from build123d import *

# Parameters (mm, degrees)
SKETCH1_R               = 1.05
SKETCH1_R_2             = 2.35
BOSS_EXTRUDE1_DEPTH     = 3
ENL_V_MAT_EXTRU_1_DEPTH = 1.5
ESQUISSE3_R             = 0.5
ESQUISSE3_R_2           = 3.75
ENL_V_MAT_EXTRU_7_DEPTH = 22.478826932


with BuildPart() as part:
    # Sketch1 → Boss-Extrude1 (new body)
    with BuildSketch(Plane(origin=(0, 0, 0), x_dir=(1, 0, 0), z_dir=(0, 1, 0))):
        with BuildLine():
            Line((15.3, 15), (12.3, 15))
            ThreePointArc((12.3, 15), (3.958234572, 13.40032808), (-3.2, 8.828273999))
            ThreePointArc((-3.2, 8.828273999), (-7, 0), (-3.2, -8.828273999))
            ThreePointArc((-3.2, -8.828273999), (3.958234572, -13.40032808), (12.3, -15))
            Line((12.3, -15), (15.3, -15))
            Line((15.3, -15), (15.3, 15))
        make_face()
        with Locations(Location((13.8, -10, 0), (0, 0, 270))):
            Circle(SKETCH1_R, mode=Mode.SUBTRACT)
        with Locations(Location((13.8, 10, 0), (0, 0, 270))):
            Circle(SKETCH1_R, mode=Mode.SUBTRACT)
        with Locations(Location((0, 0, 0), (0, 0, 270))):
            Circle(SKETCH1_R_2, mode=Mode.SUBTRACT)
    extrude(amount=-BOSS_EXTRUDE1_DEPTH)

    # Esquisse1 → Enlèv. mat.-Extru.1 (cut)
    with BuildSketch(Plane(origin=(0, 0, 0), x_dir=(1, 0, 0), z_dir=(0, 1, 0))):
        with BuildLine():
            Line((2.494493937, -2.8), (14.131406802, -1.932309126))
            add(Edge.make_bspline(
                [(14.131406802, -1.932309126), (14.497286128, -1.904835216), (14.827491954, -1.746052706), (15.157338026, -1.587443187), (15.407154881, -1.318584734), (15.656200737, -1.050556048), (15.790562016, -0.709168668), (15.92490372, -0.367831024), (15.925, 0), (15.925095847, 0.366175279), (15.791018176, 0.708007672), (15.657374187, 1.048734388), (15.407835717, 1.317851242), (15.159067388, 1.586137532), (14.828615817, 1.74551148), (14.498449498, 1.904747853), (14.131406802, 1.932309126)],
                knots=[0, 0, 0, 0.125, 0.125, 0.25, 0.25, 0.375, 0.375, 0.5, 0.5, 0.625, 0.625, 0.75, 0.75, 0.875, 0.875, 1, 1, 1], degree=2))
            Line((14.131406802, 1.932309126), (2.494493937, 2.8))
            ThreePointArc((2.494493937, 2.8), (-3.75, 0), (2.494493937, -2.8))
        make_face()
    extrude(amount=-ENL_V_MAT_EXTRU_1_DEPTH, mode=Mode.SUBTRACT)

    # Esquisse3 → Enlèv. mat.-Extru.7 (cut, through all)
    with BuildSketch(Plane(origin=(0, -1.5, 0), x_dir=(1, 0, 0), z_dir=(0, 1, 0))):
        with Locations(Location((4.9, 0, 0), (0, 0, 270))):
            Circle(ESQUISSE3_R)
        with Locations(Location((6.9, 0, 0), (0, 0, 270))):
            Circle(ESQUISSE3_R)
        with Locations(Location((8.9, 0, 0), (0, 0, 270))):
            Circle(ESQUISSE3_R)
        with Locations(Location((10.9, 0, 0), (0, 0, 270))):
            Circle(ESQUISSE3_R)
        with Locations(Location((12.9, 0, 0), (0, 0, 270))):
            Circle(ESQUISSE3_R)
        with Locations(Location((0, 0, 0), (0, 0, 270))):
            Circle(ESQUISSE3_R_2)
    extrude(amount=-ENL_V_MAT_EXTRU_7_DEPTH, mode=Mode.SUBTRACT)


solid = part.part
The model under review builds one solid part; all positions refer to its coordinate system, in mm. A direction names the side the tool comes from. Round coordinates to 2 decimals unless told otherwise and drop trailing zeros. Order: outer loops, then holes, each group sorted by start corner. A loop starts at its lowest first (then second) coordinate and runs counter-clockwise, first axis right, second up. Notation, with made-up numbers: (29.25, 67.25) -> (81.25, 67.25) arc R21 cw to (81.25, 85.25) -> close; hole circle Ø9 at (-8.75, 71). An arc over 180 degrees is marked (long way). Return JSON: item names as keys, results as strings.
1. Take a section at C-C (z = 10). Write out the cut boundary in (x, y), then the cut area to 3 significant figures.
Answer block:
{"outline": "(-1.86, -3) -> (12.75, -3) -> (12.75, 0) -> (-1.86, 0) -> close; (14.85, -3) -> (15.3, -3) -> (15.3, 0) -> (14.85, 0) -> close", "area": "45.2 mm²"}
2. Take a section at B-B (x = 13.8). Write out the cut boundary in (y, z).
Answer block:
{"outline": "(-3, -15) -> (0, -15) -> (0, -11.05) -> (-3, -11.05) -> close; (-3, -8.95) -> (0, -8.95) -> (0, -1.96) -> (-1.5, -1.96) -> (-1.5, 1.96) -> (0, 1.96) -> (0, 8.95) -> (-3, 8.95) -> close; (-3, 11.05) -> (0, 11.05) -> (0, 15) -> (-3, 15) -> close"}
3. Take a section at D-D (x = 10.9). Write out the cut boundary in (y, z), then the cut area to 3 significant figures.
Answer block:
{"outline": "(-3, -14.96) -> (0, -14.96) -> (0, -2.17) -> (-1.5, -2.17) -> (-1.5, -0.5) -> (-3, -0.5) -> close; (-3, 0.5) -> (-1.5, 0.5) -> (-1.5, 2.17) -> (0, 2.17) -> (0, 14.96) -> (-3, 14.96) -> close", "area": "81.7 mm²"}
4. Insertion check: P1, Ø1, axis at x = 6, y = -2, coming from the -Z side; P2, Ø8.5, axis at x = 0, z = 0, coming from the +Y side; P3, Ø1.5, axis at y = -1.5, z = -1.5, coming from the -X side; P4, Ø1, axis at x = -3, y = -1, coming from the -Z side. Each pin has a flat end and moves straight along its axis. Give the tip position at first contact, or say it passes through.
Answer block:
{"P1": "stops at z = -14.24", "P2": "stops at y = 0", "P3": "stops at x = -6.98", "P4": "stops at z = -9.46"}
5. For L1, parallel to Z at x = 12.25, y = -1.4; L2, parallel to Y at x = 7.5, z = -1.5; L3, parallel to Z at x = 4.5, y = -2.55, list the stretches that pass through material, from the lowest coordinate up. Write a range as [from, to].
Answer block:
{"L1": "z = [-15, -2.07], [2.07, 15]", "L2": "y = [-3, -1.5]", "L3": "z = [-13.61, -0.3], [0.3, 13.61]"}
6. Take a section at A-A (y = -1.9). State how many separate pieces and enclosed holes the cut face has, then the cut area to 3 significant figures.
Answer block:
{"separate pieces": "1", "enclosed holes": "8", "area": "486 mm²"}
7. The part is to be moulded in two halves that separate along X. For faces 3 (the face through (14.12, -1.48, 11)), 4 (the face through (14, -1, 15)), 5 (the face through (3.847, -1.479, 13.356)), say which applies: +X half, -X half, draft (parallel to the pull), parting line (faces both ways), or undercut.
Answer block:
{"face 3": "undercut", "face 4": "draft", "face 5": "-X half"}
8. For faces 1 (the face through (9, -1.5, 1)), 2 (the face through (-7, -1, 0)), list the 3-axis set-ups (+Z, -Z, +X, -X, +Y, -Y) from which the entire face can be reached by the end or side of a thin tool; tool diameter is ignored.
Answer block:
{"face 1": "+Y", "face 2": "-X, +Y, -Y"}
